Solid Edge part; units mm, degrees
sketch "Sketch1" plane through (0, 0, 0) normal (1, 0, 0) x (0, 1, 0)
  line L0 (4.5, -3.175) -> (4.5, 3.175)
  line L1 (4.5, 3.175) -> (-4.5, 3.175)
  line L2 (-4.5, 3.175) -> (-4.5, -3.175)
  line L3 (-4.5, -3.175) -> (4.5, -3.175)
  line L4 (3, -1.65) -> (3, 1.65)
  line L5 (3, 1.65) -> (-3, 1.65)
  line L6 (-3, 1.65) -> (-3, -1.65)
  line L7 (-3, -1.65) -> (3, -1.65)
extrude "Protrusion1" add sketch "Sketch1" against normal blind 5
sketch "Sketch2" plane through (0, 0, 0) normal (1, 0, 0) x (0, 1, 0)
  line L0 (4.5, -3.175) -> (4.5, 3.175)
  line L1 (4.5, 3.175) -> (-4.5, 3.175)
  line L2 (-4.5, 3.175) -> (-4.5, -3.175)
  line L3 (-4.5, -3.175) -> (4.5, -3.175)
extrude "ExtrudedProtrusion_2" add sketch "Sketch2" along normal blind 15
sketch "Sketch3" plane through (2.2625, 0, 3.175) normal (0, 0, 1) x (1, 0, 0)
  circle A0 centre (7.7375, 0) radius 3.25
extrude "Cutout1" cut sketch "Sketch3" against normal up to next
fillet "Round1" radius 0.5 4 edges at (-5, 4.5, 0) (-5, -4.5, 0) (15, 4.5, 0) (15, -4.5, 0)
Design review of the part built by this model. Coordinates are the model's own, in mm. A direction names the side the tool comes from. Round coordinates to 2 decimals unless told otherwise and drop trailing zeros. Loops run counter-clockwise (first coordinate to the right, second up) from the corner with the lowest first, then second, coordinate; pieces in that order, holes last. Notation, with made-up numbers: M -22.75,-32.75 L 30.25,-32.75 A25 cw 30.25,-3.75 Z; hole C -10.5,58.5 d8. An arc over 180 degrees is marked long. Answer as a JSON object with one key per item and string values.
Item 1: The part is to be moulded in two halves that separate along Z. For faces 1 (the flat face through (5, 0, 3.175)), 2 (the flat face through (5, 4.5, 0)), 3 (the flat face through (-2, 3, 0)), say which applies: pulls with the +Z half, pulls with the -Z half, needs draft (parallel to the pull), parting line crosses it, or undercut.
Answer sheet:
{"face 1": "pulls with the +Z half", "face 2": "needs draft", "face 3": "undercut"}
Item 2: We need section D-D on x = -2.5. Give the boundary of the cut face in (y, z) (3 decimals).
Answer sheet:
{"outline": "M -4.5,-3.175 L 4.5,-3.175 L 4.5,3.175 L -4.5,3.175 Z; hole M -3,-1.65 L 3,-1.65 L 3,1.65 L -3,1.65 Z"}
Item 3: We need section B-B on z = -0.5. Give the boundary of the cut face in (x, y), and give its area (3 significant figures).
Answer sheet:
{"outline": "M -5,-4 A0.5 ccw -4.5,-4.5 L 14.5,-4.5 A0.5 ccw 15,-4 L 15,4 A0.5 ccw 14.5,4.5 L -4.5,4.5 A0.5 ccw -5,4 L -5,3 L 0,3 L 0,-3 L -5,-3 Z; hole C 10,0 d6.5", "area": "117 mm^2"}
Item 4: We need section A-A on y = 0. Give the boundary of the cut face in (x, z) (3 decimals).
Answer sheet:
{"outline": "M -5,-3.175 L 6.75,-3.175 L 6.75,3.175 L -5,3.175 L -5,1.65 L 0,1.65 L 0,-1.65 L -5,-1.65 Z; M 13.25,-3.175 L 15,-3.175 L 15,3.175 L 13.25,3.175 Z"}
Item 5: We need section C-C on x = 10. Give the boundary of the cut face in (y, z) (3 decimals), and give its area (3 significant figures).
Answer sheet:
{"outline": "M -4.5,-3.175 L -3.25,-3.175 L -3.25,3.175 L -4.5,3.175 Z; M 3.25,-3.175 L 4.5,-3.175 L 4.5,3.175 L 3.25,3.175 Z", "area": "15.9 mm^2"}
Item 6: Clearance check with a flat-ended pin moving along its axis: P1, Ø1.6, axis at y = -1, z = -0.5, coming from the -X side. State where the tip first meets the part, or that it passes through.
Answer sheet:
{"P1": "stops at x = 0"}
Item 7: Machinability: for faces 4 (the flat face through (-2, -3, 0)), 5 (the flat face through (15, 0, 0)), which of the approach directions +Z, -Z, +X, -X, +Y, -Y give a long, thin tool a straight path to every point of the face, cutting with its end or side? Answer none if there is none.
Answer sheet:
{"face 4": "-X", "face 5": "+Z, -Z, +X, +Y, -Y"}
Item 8: Wall thickness on L1, parallel to Z at x = -2.25, y = 2.75 (3 decimals); L2, parallel to Y at x = 10, z = 1.5; L3, parallel to Y at x = 8.75, z = 1.75: over which ranges is each line inside the solid? List them lowest first. Write a range as from..to.
Answer sheet:
{"L1": "z = -3.175..-1.65, 1.65..3.175", "L2": "y = -4.5..-3.25, 3.25..4.5", "L3": "y = -4.5..-3, 3..4.5"}
